```python
from build123d import *

# Parameters (mm, degrees)
SKETCH1_W           = 15.24
SKETCH1_H           = 20.8788
SKETCH1_W_2         = 10.668
SKETCH1_H_2         = 15.748
BOSS_EXTRUDE1_DEPTH = 10.16
SKETCH2_R           = 0.25
CUT_EXTRUDE1_DEPTH  = 16.24
SKETCH3_W           = 11.43
SKETCH3_H           = 17.0688
CUT_EXTRUDE2_DEPTH  = 9.652
SKETCH5_W           = 15.24
SKETCH5_H           = 20.8788
SKETCH5_W_2         = 12.24
SKETCH5_H_2         = 17.8788
CUT_EXTRUDE4_DEPTH  = 1
FILLET1_R           = 0.5


with BuildPart() as part:
    # Sketch1 → Boss-Extrude1 (new body)
    with BuildSketch(Plane(origin=(0, 0, 0), x_dir=(1, 0, 0), z_dir=(0, 1, 0))):
        with Locations((7.62, 10.4394)):
            Rectangle(SKETCH1_W, SKETCH1_H)
        with Locations((7.62, 10.4394)):
            Rectangle(SKETCH1_W_2, SKETCH1_H_2, mode=Mode.SUBTRACT)
    extrude(amount=BOSS_EXTRUDE1_DEPTH)

    # Sketch2 → Cut-Extrude1 (cut, through all)
    with BuildSketch(Plane(origin=(15.24, 0, 0), x_dir=(0, 0, -1), z_dir=(1, 0, 0))):
        with Locations((10.4394, 7.62)):
            Circle(SKETCH2_R)
    extrude(amount=-CUT_EXTRUDE1_DEPTH, mode=Mode.SUBTRACT)

    # Sketch3 → Cut-Extrude2 (cut)
    with BuildSketch(Plane.XZ):
        with Locations((7.62, -10.4394)):
            Rectangle(SKETCH3_W, SKETCH3_H)
    extrude(amount=-CUT_EXTRUDE2_DEPTH, mode=Mode.SUBTRACT)

    # Sketch5 → Cut-Extrude4 (cut)
    with BuildSketch(Plane(origin=(0, 8.01, 0), x_dir=(1, 0, 0), z_dir=(0, 1, 0))):
        with Locations((7.62, 10.4394)):
            Rectangle(SKETCH5_W, SKETCH5_H)
        with Locations((7.62, 10.4394)):
            Rectangle(SKETCH5_W_2, SKETCH5_H_2, mode=Mode.SUBTRACT)
    extrude(amount=-CUT_EXTRUDE4_DEPTH, mode=Mode.SUBTRACT)

    # Fillet1
    fillet1_edges = [part.edges().sort_by_distance(p)[0] for p in [
        (15.24, 10.16, -10.4394),
        (7.62, 10.16, -20.8788),
        (0, 10.16, -10.4394),
        (0, 3.505, -20.8788),
        (15.24, 3.505, -20.8788),
        (15.24, 3.505, 0),
        (0, 3.505, 0),
        (7.62, 10.16, 0),
        (0, 9.085, -20.8788),
        (15.24, 9.085, -20.8788),
        (15.24, 9.085, 0),
        (0, 9.085, 0),
    ]]
    fillet(fillet1_edges, radius=FILLET1_R)


solid = part.part
```
Build history of the part. All positions in model axes, mm. A direction names the side the tool comes from. Give positions to 0.01 mm unless a question says otherwise; leave off trailing zeros. Loops run counter-clockwise (first coordinate to the right, second up) from the corner with the lowest first, then second, coordinate; pieces in that order, holes last. Notation, with made-up numbers: (-31.5, -12) -> (-20.5, -12) arc R17 cw to (-20.5, 0) -> close; hole circle Ø4 at (69.25, 46). An arc over 180 degrees is marked (long way). One line per question, with ' | ' between items. Start each with the question number.
1) Cut at C-C (z = -8). Give the cut face in (x, y) (3 decimals).
2) Cut at A-A (x = 6.75). Give the cut face in (y, z) (3 decimals).
3) Two-plate mould, pull along Y, no slides. Class faces 5 (the flat face through (1, 0, -11)), 6 (the flat face through (0, 3, -10)), 7 (the flat face through (7.5, 7.5, -19.379)): released by +Y, released by -Y, zero draft, split by the parting line, or undercut.
4) 3-axis set-ups, long thin cutter, end or side, ignore diameter. For faces 1 (the flat face through (1.905, 5, -11)), 2 (the flat face through (1, 8.01, -11)), 3 (the flat face through (7.5, 7.5, -1.5)), 4 (the flat face through (13.74, 7.2, -10.3)): which of +Z, -Z, +X, -X, +Y, -Y reach the whole face in a straight line?
5) Cut at B-B (y = 7.62). Give the cut face in (x, z) (3 decimals), plus the area to 3 significant figures.
6) Cut at D-D (y = 1.75). Give the cut face in (x, z) (3 decimals).
7) Pin check, flat tips, straight feed: pin 1 (1.1 mm diameter, centred on y = 7.5, z = -7.5, fed in from -X); pin 2 (2 mm diameter, centred on x = 11.5, z = -13, fed in from +Y). Stop position of each tip, or through.
8) Probe L1, parallel to X at y = 5.5, z = -11 (3 decimals); L2, parallel to Z at x = 10.25, y = 7.5 (3 decimals); L3, parallel to Z at x = 11.5, y = 9.25 (3 decimals). List the from-to ranges inside material, lowest first.
Return value:
1) outline: (0, 0) -> (1.905, 0) -> (1.905, 9.652) -> (2.286, 9.652) -> (2.286, 10.16) -> (0.5, 10.16) arc R0.5 ccw to (0, 9.66) -> (0, 8.01) -> (1.5, 8.01) -> (1.5, 7.01) -> (0, 7.01) -> close; (12.954, 9.652) -> (13.335, 9.652) -> (13.335, 0) -> (15.24, 0) -> (15.24, 7.01) -> (13.74, 7.01) -> (13.74, 8.01) -> (15.24, 8.01) -> (15.24, 9.66) arc R0.5 ccw to (14.74, 10.16) -> (12.954, 10.16) -> close
2) outline: (0, -20.879) -> (7.01, -20.879) -> (7.01, -19.379) -> (8.01, -19.379) -> (8.01, -20.879) -> (9.66, -20.879) arc R0.5 ccw to (10.16, -20.379) -> (10.16, -18.313) -> (9.652, -18.313) -> (9.652, -18.974) -> (0, -18.974) -> close; (0, -1.905) -> (9.652, -1.905) -> (9.652, -2.565) -> (10.16, -2.565) -> (10.16, -0.5) arc R0.5 ccw to (9.66, 0) -> (8.01, 0) -> (8.01, -1.5) -> (7.01, -1.5) -> (7.01, 0) -> (0, 0) -> close
3) face 5: released by -Y | face 6: zero draft | face 7: undercut
4) face 1: -Y | face 2: none | face 3: +Z, +X, -X | face 4: +Z, -Z, +X
5) outline: (1.5, -19.379) -> (13.74, -19.379) -> (13.74, -10.689) -> (13.335, -10.689) -> (13.335, -18.974) -> (1.905, -18.974) -> (1.905, -10.689) -> (1.5, -10.689) -> close; (1.5, -10.189) -> (1.905, -10.189) -> (1.905, -1.905) -> (13.335, -1.905) -> (13.335, -10.189) -> (13.74, -10.189) -> (13.74, -1.5) -> (1.5, -1.5) -> close | area: 23.3 mm^2
6) outline: (0, -20.379) arc R0.5 ccw to (0.5, -20.879) -> (14.74, -20.879) arc R0.5 ccw to (15.24, -20.379) -> (15.24, -0.5) arc R0.5 ccw to (14.74, 0) -> (0.5, 0) arc R0.5 ccw to (0, -0.5) -> close; hole (1.905, -18.974) -> (13.335, -18.974) -> (13.335, -1.905) -> (1.905, -1.905) -> close
7) pin 1: x = 0 | pin 2: through
8) L1: 0 to 1.905, 13.335 to 15.24 | L2: -19.379 to -18.974, -1.905 to -1.5 | L3: -20.879 to -18.974, -1.905 to 0
